from build123d import *

# Parameters (mm, degrees)
SKETCH1_R               = 8
BOSS_EXTRUDE1_DEPTH     = 7.1
SKETCH2_R               = 6.11
BOSS_EXTRUDE2_DEPTH     = 7.14
SKETCH5_R               = 2.5
CUT_EXTRUDE2_DEPTH      = 16
SKETCH8_R               = 8
BOSS_EXTRUDE4_DEPTH     = 1.5
SKETCH9_R               = 2.5
CUT_EXTRUDE4_DEPTH      = 15.74
SKETCH10_W              = 16
SKETCH10_H              = 6
CUT_EXTRUDE5_DEPTH      = 10
CUT_EXTRUDE5_DEPTH_BACK = 10


with BuildPart() as part:
    # Sketch1 → Boss-Extrude1 (new body)
    with BuildSketch(Plane(origin=(0, 0, 0), x_dir=(1, 0, 0), z_dir=(0, 1, 0))):
        Circle(SKETCH1_R)
    extrude(amount=BOSS_EXTRUDE1_DEPTH)

    # Sketch2 → Boss-Extrude2 (add)
    with BuildSketch(Plane(origin=(0, 7.1, 0), x_dir=(1, 0, 0), z_dir=(0, 1, 0))):
        Circle(SKETCH2_R)
    extrude(amount=BOSS_EXTRUDE2_DEPTH)

    # Sketch5 → Cut-Extrude2 (cut)
    with BuildSketch(Plane.XZ):
        Circle(SKETCH5_R)
    extrude(amount=-CUT_EXTRUDE2_DEPTH, mode=Mode.SUBTRACT)

    # Sketch8 → Boss-Extrude4 (add)
    with BuildSketch(Plane(origin=(0, 14.24, 0), x_dir=(1, 0, 0), z_dir=(0, 1, 0))):
        Circle(SKETCH8_R)
    extrude(amount=BOSS_EXTRUDE4_DEPTH)

    # Sketch9 → Cut-Extrude4 (cut)
    with BuildSketch(Plane(origin=(0, 15.74, 0), x_dir=(1, 0, 0), z_dir=(0, 1, 0))):
        Circle(SKETCH9_R)
    extrude(amount=-CUT_EXTRUDE4_DEPTH, mode=Mode.SUBTRACT)

    # Sketch10 → Cut-Extrude5 (cut, two sides)
    with BuildSketch(Plane(origin=(0, 0, 0), x_dir=(0, 0, -1), z_dir=(1, 0, 0))) as cut_extrude5_sk:
        with Locations((0, 2.6)):
            Rectangle(SKETCH10_W, SKETCH10_H)
    extrude(amount=CUT_EXTRUDE5_DEPTH, mode=Mode.SUBTRACT)
    extrude(cut_extrude5_sk.sketch, amount=-CUT_EXTRUDE5_DEPTH_BACK, mode=Mode.SUBTRACT)


solid = part.part
Input: part model. Units: mm. Frame: model coordinates. A direction names the side the tool comes from. Give positions to 0.01 mm unless a question says otherwise; leave off trailing zeros. Order: outer loops, then holes, each group sorted by start corner. A loop starts at its lowest first (then second) coordinate and runs counter-clockwise, first axis right, second up. Notation, with made-up numbers: M 30,14 L 35,14 A26 ccw 35,34 Z; hole C -29,-22 d5. An arc over 180 degrees is marked long. Answer as a JSON object with one key per item and string values.
1. Ray query, line 1 (Z direction, x = 0, y = 10.25); line 2 (Y direction, x = 2.75, z = 5.5). Return the intervals inside material, ascending. Write a range as [from, to].
Result sheet:
{"line 1": "[-6.11, -2.5], [2.5, 6.11]", "line 2": "[5.6, 7.1], [14.24, 15.74]"}
2. Cut plane A-A, the plane z = 0. Output: boundary loops of the cut face in (x, y), and give its area (3 significant figures).
Result sheet:
{"outline": "M -8,5.6 L -2.5,5.6 L -2.5,15.74 L -8,15.74 L -8,14.24 L -6.11,14.24 L -6.11,7.1 L -8,7.1 Z; M 2.5,5.6 L 8,5.6 L 8,7.1 L 6.11,7.1 L 6.11,14.24 L 8,14.24 L 8,15.74 L 2.5,15.74 Z", "area": "84.6 mm²"}
3. Cut plane C-C, the plane y = 10.5. Output: boundary loops of the cut face in (x, z), and give its area (3 significant figures).
Result sheet:
{"outline": "C 0,0 d12.22; hole C 0,0 d5", "area": "97.6 mm²"}
4. Cut plane B-B, the plane x = 0. Output: boundary loops of the cut face in (y, z).
Result sheet:
{"outline": "M 5.6,-8 L 7.1,-8 L 7.1,-6.11 L 14.24,-6.11 L 14.24,-8 L 15.74,-8 L 15.74,-2.5 L 5.6,-2.5 Z; M 5.6,2.5 L 15.74,2.5 L 15.74,8 L 14.24,8 L 14.24,6.11 L 7.1,6.11 L 7.1,8 L 5.6,8 Z"}
5. Cut plane D-D, the plane x = 3. Output: boundary loops of the cut face in (y, z), and give its area (3 significant figures).
Result sheet:
{"outline": "M 5.6,-7.42 L 7.1,-7.42 L 7.1,-5.32 L 14.24,-5.32 L 14.24,-7.42 L 15.74,-7.42 L 15.74,7.42 L 14.24,7.42 L 14.24,5.32 L 7.1,5.32 L 7.1,7.42 L 5.6,7.42 Z", "area": "121 mm²"}
6. Pull-direction query (Y, two-part tool) for faces 1 (the flat face through (-2, 14.24, 6)), 2 (the cylindrical face through (-1.73, 6.34, 7.81)), 3 (the flat face through (2, 5.6, 2)); classes: +Y half, -Y half, draft (parallel to the pull), parting line (faces both ways), or undercut.
Result sheet:
{"face 1": "undercut", "face 2": "draft", "face 3": "-Y half"}
7. Reachability of faces 4 (the flat face through (-2, 7.1, 6)), 5 (the flat face through (2, 15.74, -2)) from +Z, -Z, +X, -X, +Y, -Y: full face, straight path, thin tool, end or side. Return the list, or none.
Result sheet:
{"face 4": "none", "face 5": "+Z, -Z, +X, -X, +Y"}
8. First-contact query: P1, Ø3, axis at x = -2, y = 7.5, coming from the -Z side; P2, Ø6, axis at x = 3.5, y = 11, coming from the -Z side; P3, Ø3, axis at x = 2.5, y = 11, coming from the -Z side; P4, Ø4, axis at x = 0, z = 0, coming from the -Y side. Flat tips, straight axial feed; report the tip coordinate or a pass-through.
Result sheet:
{"P1": "z = -7.98", "P2": "z = -6.09", "P3": "z = -6.03", "P4": "through"}
